from build123d import *

# Parameters (mm, degrees)
F2_R     = 2.5
F3_DEPTH = 25.4
F4_DEPTH = 3
F2_R_2   = 6
F2_R_3   = 0.5
F5_DEPTH = 1
F6_DEPTH = 1.25
F7_R     = 3
F7_R_2   = 1.75
F8_DEPTH = 8


with BuildPart() as f1:
    # F0 (on Right) → F1 (revolve)
    with BuildSketch(Plane.YZ):
        with BuildLine():
            Line((1.72323, 13), (1.72323, 15.984875))
            ThreePointArc((1.72323, 15.984875), (0, 19), (-1.72323, 15.984875))
            Line((-1.72323, 15.984875), (-1.72323, 13))
            Line((-1.72323, 13), (-0.861619, 13))
            Line((-0.861619, 13), (-0.861619, 0))
            Line((-0.861619, 0), (0.861619, 0))
            Line((0.861619, 0), (0.861619, 13))
            Line((0.861619, 13), (1.72323, 13))
        make_face()
    revolve(axis=Axis((0, 0, 0), (0, 1, 0)))

    # F2 (on face) → F3 (cut)
    with BuildSketch(Plane.XZ.offset(0.861619)):
        with Locations((0, 9.500006)):
            Circle(F2_R)
        with Locations((6.717518, 6.717518)):
            Circle(F2_R)
        with Locations((9.500006, 0)):
            Circle(F2_R)
        with Locations((6.717518, -6.717518)):
            Circle(F2_R)
        with Locations((0, -9.500006)):
            Circle(F2_R)
        with Locations((-6.717518, -6.717518)):
            Circle(F2_R)
        with Locations((-9.500006, 0)):
            Circle(F2_R)
        with Locations((-6.717518, 6.717518)):
            Circle(F2_R)
    extrude(amount=-F3_DEPTH, mode=Mode.SUBTRACT)

    # F2 (on face) → F4 (join)
    with BuildSketch(Plane.XZ.offset(0.861619)):
        Circle(F2_R)
    extrude(amount=F4_DEPTH)

    # F2 (on face) → F5 (join)
    with BuildSketch(Plane.XZ.offset(0.861619)):
        Circle(F2_R_2)
        with Locations((-1.313321, -4.041987)):
            Circle(F2_R_3, mode=Mode.SUBTRACT)
        with Locations((-3.438319, -2.498085)):
            Circle(F2_R_3, mode=Mode.SUBTRACT)
        with Locations((1.313321, -4.041987)):
            Circle(F2_R_3, mode=Mode.SUBTRACT)
        with Locations((3.438319, -2.498085)):
            Circle(F2_R_3, mode=Mode.SUBTRACT)
        with Locations((-4.249997, 0)):
            Circle(F2_R_3, mode=Mode.SUBTRACT)
        with Locations((-3.438319, 2.498085)):
            Circle(F2_R_3, mode=Mode.SUBTRACT)
        with Locations((-1.313321, 4.041987)):
            Circle(F2_R_3, mode=Mode.SUBTRACT)
        Circle(F2_R, mode=Mode.SUBTRACT)
        with Locations((4.249997, 0)):
            Circle(F2_R_3, mode=Mode.SUBTRACT)
        with Locations((3.438319, 2.498085)):
            Circle(F2_R_3, mode=Mode.SUBTRACT)
        with Locations((1.313321, 4.041987)):
            Circle(F2_R_3, mode=Mode.SUBTRACT)
    extrude(amount=F5_DEPTH)

    # F2 (on face) → F6 (join)
    with BuildSketch(Plane.XZ.offset(0.861619)):
        with Locations((-1.313321, 4.041987)):
            Circle(F2_R_3)
        with Locations((1.313321, 4.041987)):
            Circle(F2_R_3)
        with Locations((3.438319, 2.498085)):
            Circle(F2_R_3)
        with Locations((4.249997, 0)):
            Circle(F2_R_3)
        with Locations((3.438319, -2.498085)):
            Circle(F2_R_3)
        with Locations((1.313321, -4.041987)):
            Circle(F2_R_3)
        with Locations((-1.313321, -4.041987)):
            Circle(F2_R_3)
        with Locations((-3.438319, -2.498085)):
            Circle(F2_R_3)
        with Locations((-4.249997, 0)):
            Circle(F2_R_3)
        with Locations((-3.438319, 2.498085)):
            Circle(F2_R_3)
    extrude(amount=F6_DEPTH)

    # F7 (on face) → F8 (join)
    with BuildSketch(Plane(origin=(0, 0.861619, 0), x_dir=(-1, 0, 0), z_dir=(0, 1, 0))):
        Circle(F7_R)
        Circle(F7_R_2, mode=Mode.SUBTRACT)
    extrude(amount=F8_DEPTH)


solid = f1.part
The model under review builds one solid part; all positions refer to its coordinate system, in mm. A direction names the side the tool comes from. Round coordinates to 2 decimals unless told otherwise and drop trailing zeros. Loops run counter-clockwise (first coordinate to the right, second up) from the corner with the lowest first, then second, coordinate; pieces in that order, holes last. Notation, with made-up numbers: (-5, 19.5) -> (45, 19.5) arc R18 cw to (45, 36.5) -> close; hole circle Ø10 at (62.5, -22.5). An arc over 180 degrees is marked (long way). Write item = value, one per line. Start each with the question number.
Item 1: For faces 1 (the flat face through (1, -2.112, -4)), 2 (the flat face through (-4, -2.112, 0)), 3 (the cylindrical face through (-0.54, -2.85, -2.44)), 4 (the flat face through (4, -2.112, 0)), 5 (the cylindrical face through (7.87, -0.01, 4.5)), list the 3-axis set-ups (+Z, -Z, +X, -X, +Y, -Y) from which the entire face can be reached by the end or side of a thin tool; tool diameter is ignored.
Item 2: Take a section at D-D on y = -3. Give the boundary of the cut face in (x, z), plus the area to 3 significant figures.
Item 3: Take a section at B-B on z = 0. Count the separate pieces of the cut face and the enclosed holes in it, plus the area to 3 significant figures.
Item 4: Take a section at A-A on y = 7. Give the boundary of the cut face in (x, z), plus the area to 3 significant figures.
Item 5: Mouldability with a two-part tool opening along Z and no side actions: class faces 6 (the cylindrical face through (-7.91, 1.298, -10.316)), 7 (the cylindrical face through (-8.701, -0.012, 5.196)), 8 (the flat face through (-1, -2.112, 4)) as released by +Z, released by -Z, zero draft, split by the parting line, or undercut.
Item 6: To check wall thickness, follow L1, parallel to Y at x = -5, z = 14.5; L2, parallel to X at y = 5, z = -1; L3, parallel to Y at x = 1, z = 3.5. State the ranges of each line that lie inside material, in increasing order.
Item 7: Insertion check: pin 1 (1.1 mm diameter, centred on x = 1.5, z = -4, fed in from -Y); pin 2 (6.5 mm diameter, centred on x = 6.72, z = -6.72, fed in from +Y); pin 3 (10 mm diameter, centred on x = -0.5, z = -11.5, fed in from +Y). Each pin has a flat end and moves straight along its axis. Give the tip position at first contact, or say it passes through.
Result:
q1.face_1 = -Z, +X, -X, -Y
q1.face_2 = +Z, -Z, -X, -Y
q1.face_3 = -Y
q1.face_4 = +Z, -Z, +X, -Y
q1.face_5 = +Y, -Y
q2.outline = circle Ø5 at (0, 0)
q2.area = 19.6 mm²
q3.separate_pieces = 3
q3.enclosed_holes = 0
q3.area = 111 mm²
q4.outline = circle Ø6 at (0, 0); hole circle Ø3.5 at (0, 0)
q4.area = 18.7 mm²
q5.face_6 = undercut
q5.face_7 = undercut
q5.face_8 = zero draft
q6.L1 = -1.72 to 1.72
q6.L2 = -2.83 to -1.44, 1.44 to 2.83
q6.L3 = -1.86 to 0.86
q7.pin_1 = -2.11
q7.pin_2 = 0.86
q7.pin_3 = 1.94
